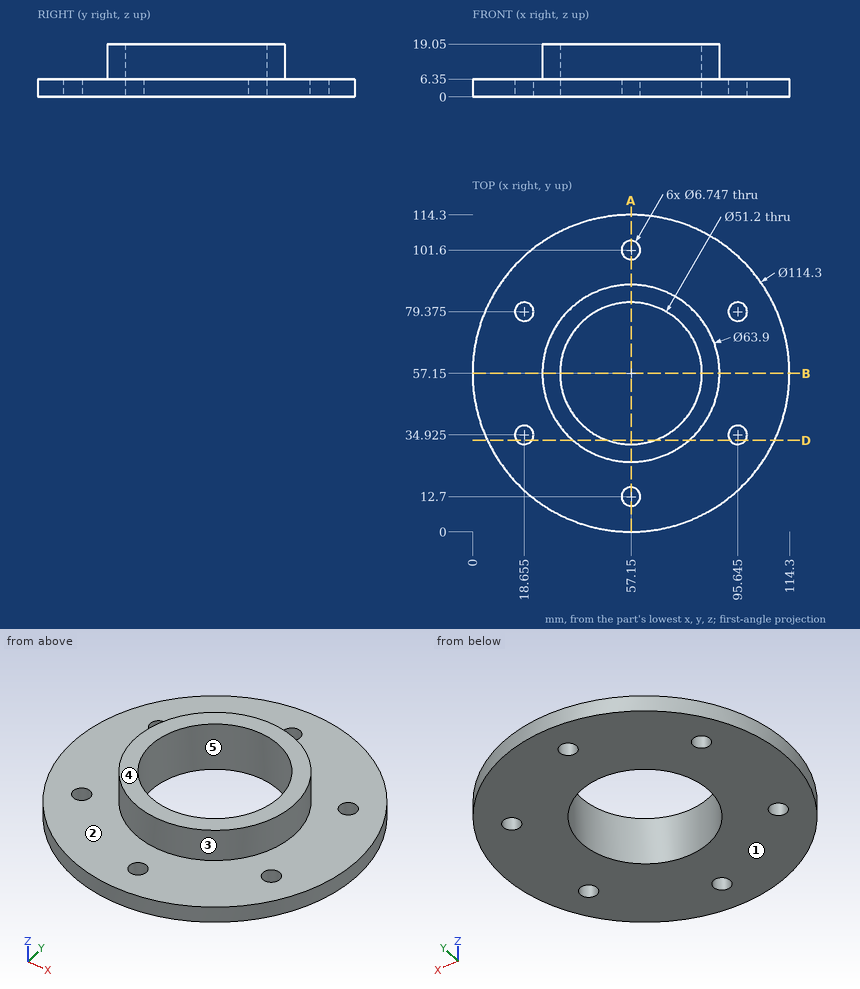
Geometry check sheet. Reference: drawing and pictorial views, mm from the part's lowest x, y, z. A direction names the side the tool comes from. Coordinates: 2 decimals unless noted, no trailing zeros. Order: outer loops, then holes, each group sorted by start corner. A loop starts at its lowest first (then second) coordinate and runs counter-clockwise, first axis right, second up. Notation, with made-up numbers: (-11.5, -26.75) - (24.5, -26.75) arc R17 ccw to (24.5, -9.75) - close; hole circle Ø10 at (56.5, 1). An arc over 180 degrees is marked (long way). Answer in a Markdown table with one row per item. Add a question column.
1) Set-up check for the marked faces 1 and 2: record each of +Z, -Z, +X, -X, +Y, -Y from which the full face is reachable in a straight line by a thin tool's end or side.
2) Release check for a two-part mould opening along X. For the marked faces 3, 4 and 5 record: +X half, -X half, draft (parallel to the pull), parting line (faces both ways), or undercut.
3) Gauge pin test, flat ends, axial feed: P1, Ø4, axis at x = 72, z = 9.5, coming from the -Y side; P2, Ø1, axis at x = 37.5, z = 17, coming from the +Y side (1 decimal); P3, Ø5, axis at x = 102.5, y = 61, coming from the +Z side. Record the tip position at first contact, or that the pin passes through.
4) Cross-section at A-A, the plane x = 57.15. Record the cut outline in (y, z), then the cut area to 3 significant figures.
5) Cross-section at D-D, the plane y = 33. State how many separate pieces and enclosed holes the cut face has, then the cut area to 3 significant figures.
6) Cross-section at B-B, the plane y = 57.15. Record the cut outline in (x, z).
7) Material ranges on line 1 along Y through (x, z) = (57.15, 5); line 2 along Y through (x, z) = (57.15, 13.5); line 3 along Y through (x, z) = (20, 3.75), recorded low to high. Write a range as [from, to].
Check result:
| question | item | result |
|---|---|---|
| 1 | face 1 | -Z, +X, -X, +Y, -Y |
| 1 | face 2 | +Z |
| 2 | face 3 | parting line |
| 2 | face 4 | draft |
| 2 | face 5 | undercut |
| 3 | P1 | stops at y = 27.9 |
| 3 | P2 | stops at y = 82.7 |
| 3 | P3 | stops at z = 6.35 |
| 4 | outline | (0, 0) - (9.33, 0) - (9.33, 6.35) - (0, 6.35) - close; (16.07, 0) - (31.55, 0) - (31.55, 19.05) - (25.2, 19.05) - (25.2, 6.35) - (16.07, 6.35) - close; (82.75, 0) - (98.23, 0) - (98.23, 6.35) - (89.1, 6.35) - (89.1, 19.05) - (82.75, 19.05) - close; (104.97, 0) - (114.3, 0) - (114.3, 6.35) - (104.97, 6.35) - close |
| 4 | area | 476 mm² |
| 5 | separate pieces | 4 |
| 5 | enclosed holes | 0 |
| 5 | area | 795 mm² |
| 6 | outline | (0, 0) - (31.55, 0) - (31.55, 19.05) - (25.2, 19.05) - (25.2, 6.35) - (0, 6.35) - close; (82.75, 0) - (114.3, 0) - (114.3, 6.35) - (89.1, 6.35) - (89.1, 19.05) - (82.75, 19.05) - close |
| 7 | line 1 | y = [0, 9.33], [16.07, 31.55], [82.75, 98.23], [104.97, 114.3] |
| 7 | line 2 | y = [25.2, 31.55], [82.75, 89.1] |
| 7 | line 3 | y = [13.72, 31.83], [38.02, 76.28], [82.47, 100.58] |
